CAD build for the part. Positions are in the model's coordinates, mm. Give positions to 0.01 mm unless a question says otherwise; leave off trailing zeros. Write each loop counter-clockwise with the first axis right and the second up, starting at its lowest first coordinate (ties: lowest second). Pieces come first, ordered by that corner, then holes. Notation, with made-up numbers: (34.25, 2) - (43.25, 2) arc R25 ccw to (43.25, 17) - close; hole circle Ø8 at (-18.5, -28). An arc over 180 degrees is marked (long way). Answer as a JSON object with one key per item and string values.
from build123d import *

# Parameters (mm, degrees)
F1_DEPTH = 9.398


with BuildPart() as f1:
    # F0 (on Front) → F1 (new body)
    with BuildSketch(Plane.XZ):
        with BuildLine():
            Line((16.137162, 43.196354), (16.137162, 34.891911))
            ThreePointArc((16.137162, 34.891911), (28.218261, 32.258096), (40.29936, 34.891911))
            Line((40.29936, 34.891911), (40.29936, 43.196354))
            ThreePointArc((40.29936, 43.196354), (28.218261, 39.441099), (16.137162, 43.196354))
        make_face()
        with BuildLine():
            ThreePointArc((40.29936, -45.501441), (28.231979, -51.583741), (16.137162, -45.556184))
            Line((16.137162, -45.556184), (16.144373, -52.855063))
            ThreePointArc((16.144373, -52.855063), (28.295737, -56.862997), (40.46179, -52.899871))
            Line((40.46179, -52.899871), (40.29936, -45.501441))
        make_face()
        with BuildLine():
            ThreePointArc((40.29936, 34.891911), (28.218261, 32.258096), (16.137162, 34.891911))
            Line((16.137162, 34.891911), (16.137162, -45.556184))
            ThreePointArc((16.137162, -45.556184), (28.231979, -51.583741), (40.29936, -45.501441))
            Line((40.29936, -45.501441), (40.29936, 34.891911))
        make_face()
    extrude(amount=F1_DEPTH)


solid = f1.part
Item 1: Flat gauge pins, fed straight in: P1, Ø5, axis at x = 38, y = -5, coming from the +Z side; P2, Ø4, axis at x = 32, y = -6, coming from the -Z side; P3, Ø1.5, axis at x = 24, y = -4.5, coming from the -Z side. Where does each tip first touch, or does it go through?
Entries:
{"P1": "z = 43.2", "P2": "z = -56.8", "P3": "z = -56.55"}
Item 2: Mould opens along X. For faces 1 (the cylindrical face through (28.11, -4.63, -56.86)), 2 (the cylindrical face through (28.4, -4.63, 39.44)), 3 (the flat face through (40.299, -5, -2)), 4 (the flat face through (28, -9.398, -6)) say: +X half, -X half, draft (parallel to the pull), parting line (faces both ways), or undercut.
Entries:
{"face 1": "parting line", "face 2": "undercut", "face 3": "+X half", "face 4": "draft"}
Item 3: Cut at B-B (x = 35.5). Give the cut face in (y, z).
Entries:
{"outline": "(-9.4, -55.57) - (0, -55.57) - (0, 40.72) - (-9.4, 40.72) - close"}
Item 4: Probe line 1 (X direction, y = -6, z = 25.5); line 2 (Z direction, x = 28, y = -7.5); line 3 (Z direction, x = 27.5, y = -4). List the from-to ranges inside material, lowest first. Write a range as from..to.
Entries:
{"line 1": "16.14..40.3", "line 2": "-56.86..39.44", "line 3": "-56.85..39.45"}
Item 5: Cut at A-A (y = -3). Give the cut face in (x, z), and give its area (3 significant figures).
Entries:
{"outline": "(16.14, -52.86) arc R20.54 ccw to (40.46, -52.9) - (40.3, -45.5) - (40.3, 43.2) arc R21.31 cw to (16.14, 43.2) - (16.14, -45.56) - close", "area": "2,330 mm2"}
Item 6: Cut at C-C (x = 19.25). Give the cut face in (y, z), and give its area (3 significant figures).
Entries:
{"outline": "(-9.4, -54.75) - (0, -54.75) - (0, 41.42) - (-9.4, 41.42) - close", "area": "904 mm2"}
